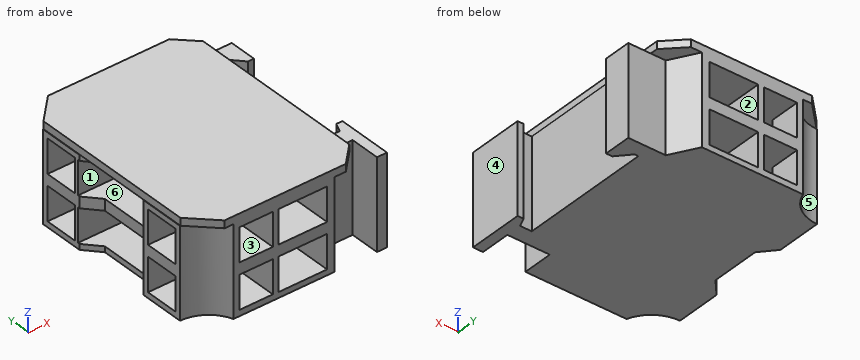
from build123d import *

# Parameters (mm, degrees)
EXTRUDE_2_DEPTH     = 24
SKETCH_4_W          = 8.901377932
SKETCH_4_H          = 8.901377932
SKETCH_4_W_2        = 13
SKETCH_4_H_2        = 9
CUT_EXTRUDE_3_DEPTH = 15
SKETCH_5_R          = 2
CUT_EXTRUDE_4_DEPTH = 2
SKETCH_6_W          = 8.901377932
SKETCH_6_H          = 8.901377932
SKETCH_6_W_2        = 13
SKETCH_6_H_2        = 9
CUT_EXTRUDE_5_DEPTH = 15
SKETCH_7_W          = 9
SKETCH_7_H          = 9
SKETCH_7_H_2        = 18.551992086
CUT_EXTRUDE_6_DEPTH = 15
EXTRUDE_3_DEPTH     = 2


with BuildPart() as part:
    # Эскиз1 → Вытянуть2 (new body)
    with BuildSketch(Plane.XY):
        with BuildLine():
            Line((53.716826077, 100.302263468), (49.716826077, 107.299731538))
            Line((49.716826077, 107.299731538), (43.716826077, 107.299731538))
            Line((43.716826077, 107.299731538), (22.716826077, 107.299731538))
            ThreePointArc((22.716826077, 107.299731538), (19.267726905, 102.594638084), (13.716826077, 100.799731538))
            Line((13.716826077, 100.799731538), (13.716826077, 88.799731538))
            Line((13.716826077, 88.799731538), (17.252144627, 84.799731538))
            Line((17.252144627, 84.799731538), (17.252144627, 71.799731538))
            Line((17.252144627, 71.799731538), (13.716826077, 67.799731538))
            Line((13.716826077, 67.799731538), (13.716826077, 55.799731538))
            ThreePointArc((13.716826077, 55.799731538), (19.267726905, 54.004824992), (22.716826077, 49.299731538))
            Line((22.716826077, 49.299731538), (49.716826077, 49.299731538))
            Line((49.716826077, 49.299731538), (49.716826077, 57.299731538))
            Line((49.716826077, 57.299731538), (61.039926278, 57.299731538))
            Line((61.039926278, 57.299731538), (61.039926278, 49.299731538))
            Line((61.039926278, 49.299731538), (63.716826077, 49.299731538))
            Line((63.716826077, 49.299731538), (63.716826077, 57.299731538))
            Line((63.716826077, 57.299731538), (63.716826077, 63.945130452))
            Line((63.716826077, 63.945130452), (62.075665924, 63.945130452))
            Line((62.075665924, 63.945130452), (61.039926278, 61.482439413))
            Line((61.039926278, 61.482439413), (57.925918002, 61.482439413))
            Line((57.925918002, 61.482439413), (57.925918002, 96.482439413))
            Line((57.925918002, 96.482439413), (58.925918002, 96.482439413))
            Line((58.925918002, 96.482439413), (62.075665924, 93.009879938))
            Line((62.075665924, 93.009879938), (63.716826077, 93.009879938))
            Line((63.716826077, 93.009879938), (63.716826077, 100.302263468))
            Line((63.716826077, 100.302263468), (53.716826077, 100.302263468))
        make_face()
    extrude(amount=EXTRUDE_2_DEPTH)

    # Эскиз4 → Вырез-Вытянуть3 (cut)
    with BuildSketch(Plane(origin=(0, 107.299731538, 0), x_dir=(-1, 0, 0), z_dir=(0, 1, 0))):
        with Locations((-28.766137111, 6.049311034)):
            Rectangle(SKETCH_4_W, SKETCH_4_H)
        with Locations((-28.766137111, 18.049311034)):
            Rectangle(SKETCH_4_W, SKETCH_4_H)
        with Locations((-41.216826077, 18)):
            Rectangle(SKETCH_4_W_2, SKETCH_4_H_2)
        with Locations((-41.216826077, 6)):
            Rectangle(SKETCH_4_W_2, SKETCH_4_H_2)
    extrude(amount=-CUT_EXTRUDE_3_DEPTH, mode=Mode.SUBTRACT)

    # Эскиз5 → Вырез-Вытянуть4 (cut)
    with BuildSketch(Plane(origin=(0, 92.299731538, 0), x_dir=(-1, 0, 0), z_dir=(0, 1, 0))):
        with Locations(Location((-41.216826077, 18, 0), (0, 0, 90))):
            Circle(SKETCH_5_R)
        with Locations(Location((-41.216826077, 6, 0), (0, 0, 90))):
            Circle(SKETCH_5_R)
    extrude(amount=-CUT_EXTRUDE_4_DEPTH, mode=Mode.SUBTRACT)

    # Эскиз6 → Вырез-Вытянуть5 (cut)
    with BuildSketch(Plane.XZ.offset(-49.299731538)):
        with Locations((28.766137111, 6.049311034)):
            Rectangle(SKETCH_6_W, SKETCH_6_H)
        with Locations((41.216826077, 6)):
            Rectangle(SKETCH_6_W_2, SKETCH_6_H_2)
        with Locations((41.216826077, 18)):
            Rectangle(SKETCH_6_W_2, SKETCH_6_H_2)
        with Locations((28.766137111, 18.049311034)):
            Rectangle(SKETCH_6_W, SKETCH_6_H)
    extrude(amount=-CUT_EXTRUDE_5_DEPTH, mode=Mode.SUBTRACT)

    # Эскиз7 → Вырез-Вытянуть6 (cut)
    with BuildSketch(Plane.ZY.offset(-13.716826077)):
        with Locations((18, 94.799731538)):
            Rectangle(SKETCH_7_W, SKETCH_7_H)
        with Locations((18, 61.799731538)):
            Rectangle(SKETCH_7_W, SKETCH_7_H)
        with Locations((6, 94.799731538)):
            Rectangle(SKETCH_7_W, SKETCH_7_H)
        with Locations((6, 61.799731538)):
            Rectangle(SKETCH_7_W, SKETCH_7_H)
        with Locations((6, 80.02885964)):
            Rectangle(SKETCH_7_W, SKETCH_7_H_2)
        with Locations((18, 80.02885964)):
            Rectangle(SKETCH_7_W, SKETCH_7_H_2)
    extrude(amount=-CUT_EXTRUDE_6_DEPTH, mode=Mode.SUBTRACT)

    # Эскиз8 → Вытянуть3 (add)
    with BuildSketch(Plane.XY.offset(24)):
        Polygon((20.331732254, 49.299731538), (52.716931495, 49.299731538), (57.716931495, 54.299731538), (57.716931495, 102.299731538), (52.716931495, 107.299731538), (20.331732254, 107.299731538), (13.831732254, 100.799731538), (13.831732254, 55.799731538), align=None)
    extrude(amount=EXTRUDE_3_DEPTH)


solid = part.part
The listing builds one solid part. Answer for the finished solid, in the listing's coordinates (mm). Face numbers are marked on the shaded views. A direction names the side the tool comes from. Coordinates: 2 decimals unless noted, no trailing zeros. Loops run counter-clockwise (first coordinate to the right, second up) from the corner with the lowest first, then second, coordinate; pieces in that order, holes last. Notation, with made-up numbers: (53.25, -20) -> (62.25, -20) arc R22 cw to (62.25, 1) -> close; hole circle Ø2 at (17.5, 62.25). An arc over 180 degrees is marked (long way). Write item = value, one per line. Start each with the question number.
1) A tool of negligible diameter and unlimited length cuts with its end or side. For the marked faces 1, 2 and 3, from which of +Z, -Z, +X, -X, +Y, -Y can it reach the whole face along a straight path? Write none if from no direction.
2) Given pin 1 Ø5 at (x, z) = (54.5, 7.5) entering from +Y; pin 2 Ø1.5 at (x, z) = (40.5, 16.5) entering from +Y; pin 3 Ø10 at (y, z) = (76.5, 6) entering from -X, each flat-ended and moving along its own axis, determine where each tip first touches the part or whether it passes through.
3) Straight lines are drawn through the part: line 1 (Y direction, x = 23, z = 20.5); line 2 (Z direction, x = 43, y = 97); line 3 (X direction, y = 91.65, z = 6). For each, find the intervals that lie inside material, in ascending order. Write a range as from..to.
4) The mould has two halves that part along Y. Classify the marked faces 4, 5 and 6: released by +Y, released by -Y, zero draft, split by the parting line, or undercut.
5) A cutting plane is placed at A-A (y = 63). Count the separate pieces of the cut face and the enclosed holes in it, then the cut area to 3 significant figures.
6) A cutting plane is placed at B-B (x = 44.5). Give the vertices of the cut face in (y, z).
7) A cutting plane is placed at D-D (y = 70). Give the vertices of the cut face in (x, z).
Responses:
q1.face_1 = -X
q1.face_2 = +Y
q1.face_3 = -Y
q2.pin_1 = 103.31
q2.pin_2 = 92.3
q2.pin_3 = 17.25
q3.line_1 = 49.3..57.3, 66.3..70.75, 89.3..90.3, 99.3..107.3
q3.line_2 = 0..1.5, 10.5..13.5, 22.5..26
q3.line_3 = 28.72..39.22, 43.22..57.93
q4.face_4 = zero draft
q4.face_5 = released by +Y
q4.face_6 = undercut
q5.separate_pieces = 2
q5.enclosed_holes = 2
q5.area = 614 mm²
q6.outline = (49.3, 0) -> (107.3, 0) -> (107.3, 1.5) -> (92.3, 1.5) -> (92.3, 10.5) -> (107.3, 10.5) -> (107.3, 13.5) -> (92.3, 13.5) -> (92.3, 22.5) -> (107.3, 22.5) -> (107.3, 26) -> (49.3, 26) -> (49.3, 22.5) -> (64.3, 22.5) -> (64.3, 13.5) -> (49.3, 13.5) -> (49.3, 10.5) -> (64.3, 10.5) -> (64.3, 1.5) -> (49.3, 1.5) -> close
q7.outline = (13.83, 24) -> (15.66, 24) -> (15.66, 0) -> (57.93, 0) -> (57.93, 24) -> (57.72, 24) -> (57.72, 26) -> (13.83, 26) -> close
